For this review, take the finished solid that the model builds, in its own axes (mm). Face numbers are marked on the shaded views. A direction names the side the tool comes from. Round coordinates to 2 decimals unless told otherwise and drop trailing zeros. Order: outer loops, then holes, each group sorted by start corner. A loop starts at its lowest first (then second) coordinate and runs counter-clockwise, first axis right, second up. Notation, with made-up numbers: (16.5, -8) - (43.5, -8) arc R7 cw to (43.5, -4) - close; hole circle Ø8 at (-7, 69). An arc over 180 degrees is marked (long way). Write each question's results on one line, items separated by ' | '. Start each with the question number.
(1) Insertion check: pin 1 Ø2.5 at (x, y) = (11.5, -5) entering from +Z (3 decimals); pin 2 Ø2 at (y, z) = (-3.5, 7.5) entering from -X; pin 3 Ø0.6 at (y, z) = (-2, 1) entering from -X. Each pin has a flat end and moves straight along its axis. Give the tip position at first contact, or say it passes through.
(2) Draft analysis for pull direction Z (two halves, no side actions). For the marked faces 1, 2 and 3, state which applies: pulls with the +Z half, pulls with the -Z half, needs draft (parallel to the pull), parting line crosses it, or undercut.
(3) For the marked faces 4, 5, 6 and 7, list the 3-axis set-ups (+Z, -Z, +X, -X, +Y, -Y) from which the entire face can be reached by the end or side of a thin tool; tool diameter is ignored.
(4) Take a section at A-A, the plane x = -6.5. Give the boundary of the cut face in (y, z).
(5) Take a section at C-C, the plane z = 12. Give the boundary of the cut face in (x, y), plus the area to 3 significant figures.
(6) Take a section at B-B, the plane x = 9.5. Give the boundary of the cut face in (y, z) (3 decimals), plus the area to 3 significant figures.
(7) For L1, parallel to X at y = -5.5, z = 5.25; L2, parallel to Z at x = 13.25, y = -2.75 (3 decimals); L3, parallel to X at y = -0.75, z = 5, list the stretches that pass through material, from the lowest coordinate up. Write a range as from..to.
```python
from build123d import *

# Parameters (mm, degrees)
F1_DEPTH = 7.366


with BuildPart() as f1:
    # F0 (on Front) → F1 (new body)
    with BuildSketch(Plane.XZ):
        with BuildLine():
            Line((-2.213933, 12.954), (-8.128, 12.954))
            ThreePointArc((-8.128, 12.954), (-8.384689, 12.935373), (-8.636, 12.879884))
            Line((-8.636, 12.879884), (-8.636, 9.144))
            Line((-8.636, 9.144), (-7.079154, 9.144))
            ThreePointArc((-7.079154, 9.144), (-6.365658, 8.785324), (-6.227896, 7.998719))
            Line((-6.227896, 7.998719), (-8.253652, 1.27))
            Line((-8.253652, 1.27), (-6.907021, 1.27))
            Line((-6.907021, 1.27), (-4.726952, 8.511281))
            ThreePointArc((-4.726952, 8.511281), (-4.406018, 8.968497), (-3.875693, 9.144))
            Line((-3.875693, 9.144), (-3.648131, 9.144))
            ThreePointArc((-3.648131, 9.144), (-3.304393, 8.971202), (-3.238025, 8.592243))
            Line((-3.238025, 8.592243), (-5.442468, 1.27))
            Line((-5.442468, 1.27), (-4.095837, 1.27))
            Line((-4.095837, 1.27), (-1.817051, 8.839178))
            ThreePointArc((-1.817051, 8.839178), (-1.662436, 9.059449), (-1.406944, 9.144))
            Line((-1.406944, 9.144), (-0.917281, 9.144))
            ThreePointArc((-0.917281, 9.144), (-0.054535, 8.992989), (0.705625, 8.557913))
            Line((0.705625, 8.557913), (5.316478, 4.728173))
            ThreePointArc((5.316478, 4.728173), (6.836798, 3.858021), (8.562289, 3.556))
            Line((8.562289, 3.556), (10.439335, 3.556))
            Line((10.439335, 3.556), (16.51, 3.556))
            Line((16.51, 3.556), (16.51, 8.382))
            ThreePointArc((16.51, 8.382), (16.286815, 8.920815), (15.748, 9.144))
            Line((15.748, 9.144), (15.494, 9.144))
            ThreePointArc((15.494, 9.144), (14.955185, 8.920815), (14.732, 8.382))
            Line((14.732, 8.382), (14.732, 6.477))
            ThreePointArc((14.732, 6.477), (14.508815, 5.938185), (13.97, 5.715))
            Line((13.97, 5.715), (10.439335, 5.715))
            Line((10.439335, 5.715), (8.941661, 5.715))
            ThreePointArc((8.941661, 5.715), (6.912095, 6.138042), (5.220557, 7.336708))
            Line((5.220557, 7.336708), (1.507171, 11.332292))
            ThreePointArc((1.507171, 11.332292), (0.805397, 11.959345), (0, 12.446188))
            ThreePointArc((0, 12.446188), (-1.078221, 12.82542), (-2.213933, 12.954))
        make_face()
        with BuildLine():
            Line((-8.636, 9.144), (-8.636, 12.879884))
            ThreePointArc((-8.636, 12.879884), (-9.553571, 12.238558), (-9.906, 11.176))
            Line((-9.906, 11.176), (-9.906, 9.144))
            Line((-9.906, 9.144), (-8.636, 9.144))
        make_face()
        Polygon((-6.907021, 1.27), (-8.253652, 1.27), (-8.636, 1.27), (-8.636, 0), (0, 0), (0, 1.27), (-4.095837, 1.27), (-5.442468, 1.27), align=None)
    extrude(amount=F1_DEPTH)


solid = f1.part
```
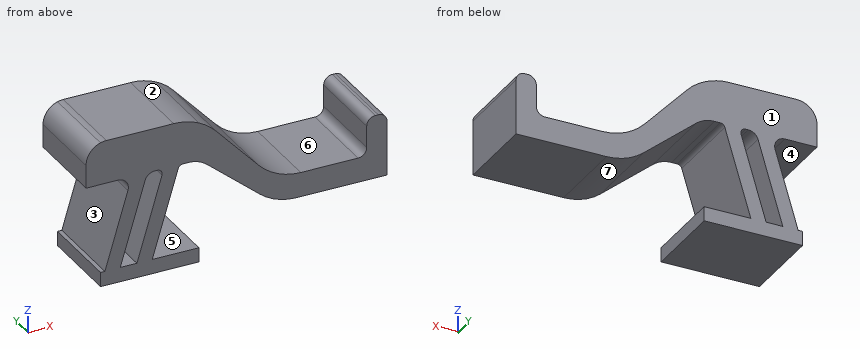
Results below:
1) pin 1: stops at z = 5.715 | pin 2: stops at x = -6.68 | pin 3: stops at x = -8.64
2) face 1: needs draft | face 2: pulls with the +Z half | face 3: undercut
3) face 4: -X, +Y, -Y | face 5: +X, +Y, -Y | face 6: +Z, +Y, -Y | face 7: -Z, +Y, -Y
4) outline: (-7.37, 0) - (0, 0) - (0, 1.27) - (-7.37, 1.27) - close; (-7.37, 2.62) - (0, 2.62) - (0, 7.09) - (-7.37, 7.09) - close; (-7.37, 8.93) - (0, 8.93) - (0, 12.95) - (-7.37, 12.95) - close
5) outline: (-9.7, -7.37) - (0.75, -7.37) - (0.75, 0) - (-9.7, 0) - close | area: 77.0 mm^2
6) outline: (-7.366, 3.556) - (0, 3.556) - (0, 5.715) - (-7.366, 5.715) - close | area: 15.9 mm^2
7) L1: x = -7.06..-5.71, -4.24..-2.9, 4.69..16.51 | L2: z = 3.556..5.715 | L3: x = -7.13..-5.78, -4.32..-2.97, 4.99..16.51
